Part model, mm, in its own coordinate system. Round coordinates to 2 decimals unless told otherwise and drop trailing zeros. Order: outer loops, then holes, each group sorted by start corner. A loop starts at its lowest first (then second) coordinate and runs counter-clockwise, first axis right, second up. Notation, with made-up numbers: (10.5, 7) -> (43.5, 7) arc R16 ccw to (43.5, 29) -> close; hole circle Ø9 at (15, 2). An arc over 180 degrees is marked (long way). Answer as a JSON object with one key per item and string values. Group by question number.
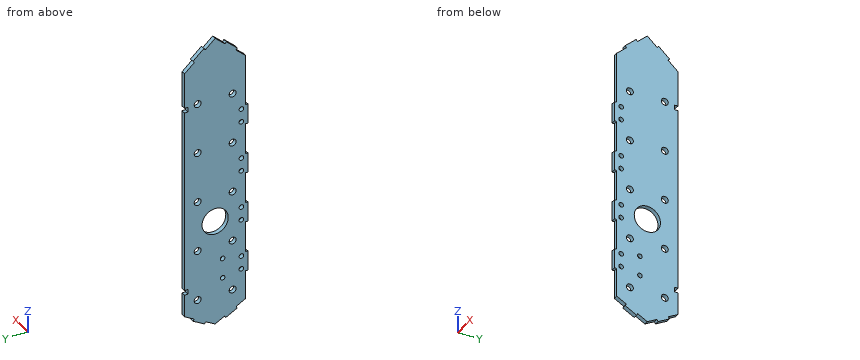
```python
from build123d import *

# Parameters (mm, degrees)
SKETCH1_W                   = 558.8
SKETCH1_H                   = 88.9
BOSS_EXTRUDE1_DEPTH         = 6.35
BOSS_EXTRUDE2_DEPTH         = 6.35
F_3_8_CLEARANCE_HOLE2_D     = 10.0838
F_3_8_CLEARANCE_HOLE3_D     = 10.0838
F_3_8_CLEARANCE_HOLE3_DEPTH = 12.7
F_3_8_CLEARANCE_HOLE3_TIP   = 3.029479155
SKETCH9_W                   = 239.47208483
SKETCH9_H                   = 88.9
CUT_EXTRUDE1_DEPTH          = 322.947408556
BOSS_EXTRUDE3_DEPTH         = 6.35
BOSS_EXTRUDE4_DEPTH         = 6.35
SKETCH12_R                  = 19.05
CUT_EXTRUDE2_DEPTH          = 322.947408556
SKETCH13_W                  = 6.858
SKETCH13_H                  = 5.2705
SKETCH13_W_2                = 6.35
SKETCH13_H_2                = 4.7625
CUT_EXTRUDE3_DEPTH          = 322.947408556
F_1_4_CLEARANCE_HOLE1_D     = 6.7564
F_1_4_CLEARANCE_HOLE2_D     = 6.7564
SKETCH18_W                  = 28.575
SKETCH18_H                  = 3.175
BOSS_EXTRUDE5_DEPTH         = 6.35


with BuildPart() as part:
    # Sketch1 → Boss-Extrude1 (new body)
    with BuildSketch(Plane(origin=(0, 0, 0), x_dir=(0, 0, -1), z_dir=(1, 0, 0))):
        Rectangle(SKETCH1_W, SKETCH1_H)
    extrude(amount=BOSS_EXTRUDE1_DEPTH)

    # Sketch2 → Boss-Extrude2 (add)
    with BuildSketch(Plane(origin=(6.35, 0, 0), x_dir=(0, 0, -1), z_dir=(1, 0, 0))):
        Polygon((-279.4, 44.45), (-318.800892213, 0), (-279.4, -44.45), align=None)
        Polygon((279.4, 44.45), (318.800892213, 0), (279.4, -44.45), align=None)
    extrude(amount=-BOSS_EXTRUDE2_DEPTH)

    # 3/8 Clearance Hole2 (through all)
    with Locations(Plane(origin=(6.35, 0, 0), x_dir=(0, 0, -1), z_dir=(1, 0, 0))):
        with Locations((-155.575, -25.4), (-155.575, 25.4), (-228.6, 25.4), (-228.6, -25.4)):
            Hole(F_3_8_CLEARANCE_HOLE2_D / 2)

    # 3/8 Clearance Hole3
    with Locations(Plane.ZY):
        with Locations((-63.5, 25.4), (-63.5, -25.4), (9.525, -25.4), (9.525, 25.4), (82.55, 25.4), (82.55, -25.4)):
            Hole(F_3_8_CLEARANCE_HOLE3_D / 2, depth=F_3_8_CLEARANCE_HOLE3_DEPTH)
            with Locations((0, 0, -(F_3_8_CLEARANCE_HOLE3_DEPTH + F_3_8_CLEARANCE_HOLE3_TIP / 2))):  # 118° drill point
                Cone(0, F_3_8_CLEARANCE_HOLE3_D / 2, F_3_8_CLEARANCE_HOLE3_TIP, mode=Mode.SUBTRACT)

    # Sketch9 → Cut-Extrude1 (cut, through all)
    with BuildSketch(Plane(origin=(6.35, 0, 0), x_dir=(0, 0, -1), z_dir=(1, 0, 0))):
        with Locations((202.286042415, 0)):
            Rectangle(SKETCH9_W, SKETCH9_H)
    extrude(amount=-CUT_EXTRUDE1_DEPTH, mode=Mode.SUBTRACT)

    # Sketch10 → Boss-Extrude3 (add)
    with BuildSketch(Plane(origin=(6.35, 0, 0), x_dir=(0, 0, -1), z_dir=(1, 0, 0))):
        Polygon((82.55, -44.45), (106.963898899, 0), (82.55, 44.45), align=None)
    extrude(amount=-BOSS_EXTRUDE3_DEPTH)

    # Sketch11 → Boss-Extrude4 (add)
    with BuildSketch(Plane.ZY):
        Polygon((-90.1923834, 30.535633289), (-92.975256742, 32.064109969), (-102.104388841, 15.442843391), (-99.321515499, 13.914366711), align=None)
        Polygon((-99.321515499, -13.914366711), (-102.104388841, -15.442843391), (-92.975256742, -32.064109969), (-90.1923834, -30.535633289), align=None)
        Polygon((292.036372489, 30.194313755), (294.412320197, 32.300375837), (308.540467431, 16.361748326), (306.164519724, 14.255686245), align=None)
        Polygon((306.164519724, -14.255686245), (308.540467431, -16.361748326), (294.412320197, -32.300375837), (292.036372489, -30.194313755), align=None)
    extrude(amount=-BOSS_EXTRUDE4_DEPTH)

    # Sketch12 → Cut-Extrude2 (cut, through all)
    with BuildSketch(Plane.ZY):
        with Locations((46.0375, 0)):
            Circle(SKETCH12_R)
    extrude(amount=-CUT_EXTRUDE2_DEPTH, mode=Mode.SUBTRACT)

    # Sketch13 → Cut-Extrude3 (cut, through all)
    with BuildSketch(Plane.ZY):
        with Locations((224.63125, 42.06875)):
            Rectangle(SKETCH13_W, SKETCH13_H)
        with Locations((224.63125, 42.06875)):
            Rectangle(SKETCH13_W_2, SKETCH13_H_2, mode=Mode.SUBTRACT)
        with Locations((-46.83125, 42.06875)):
            Rectangle(SKETCH13_W, SKETCH13_H)
        with Locations((-46.83125, 42.06875)):
            Rectangle(SKETCH13_W_2, SKETCH13_H_2, mode=Mode.SUBTRACT)
    extrude(amount=-CUT_EXTRUDE3_DEPTH, mode=Mode.SUBTRACT)


with BuildPart() as body_2:
    # of the pieces the cut leaves, the one that is kept (cut_extrude3_keep)
    add(part.part.solids().sort_by_distance((6.35, 44.45, 228.06025))[0])

    # 1/4 Clearance Hole1 (through all)
    with Locations(Plane.ZY):
        with Locations((-41.3385, -10.795), (-12.6365, -10.795)):
            Hole(F_1_4_CLEARANCE_HOLE1_D / 2)

    # 1/4 Clearance Hole2 (through all)
    with Locations(Plane.ZY):
        with Locations((-36.5125, -38.1), (-17.4625, -38.1), (36.5125, -38.1), (55.5625, -38.1), (109.5375, -38.1), (128.5875, -38.1), (182.5625, -38.1), (201.6125, -38.1)):
            Hole(F_1_4_CLEARANCE_HOLE2_D / 2)

    # Sketch18 → Boss-Extrude5 (add)
    with BuildSketch(Plane.ZY):
        with Locations((-26.9875, -46.0375)):
            Rectangle(SKETCH18_W, SKETCH18_H)
        with Locations((46.0375, -46.0375)):
            Rectangle(SKETCH18_W, SKETCH18_H)
        with Locations((119.0625, -46.0375)):
            Rectangle(SKETCH18_W, SKETCH18_H)
        with Locations((192.0875, -46.0375)):
            Rectangle(SKETCH18_W, SKETCH18_H)
    extrude(amount=-BOSS_EXTRUDE5_DEPTH)


solid = body_2.part
```
Q1. Drop flat-ended pins along their axis: pin 1 Ø3.5 at (x, y) = (4, -46.5) entering from +Z (3 decimals); pin 2 Ø1 at (x, y) = (4, -22.5) entering from +Z; pin 3 Ø2.5 at (x, y) = (2.5, -45.5) entering from +Z. Give the stop position or say it passes through.
Q2. Band-saw the part on D-D (z = -63). List the corners of the cut face in (x, y), plus the area to 3 significant figures.
Q3. Band-saw the part on C-C (y = -25.4). List the corners of the cut face in (x, z), plus the area to 3 significant figures.
Q4. Band-saw the part on A-A (z = 82.55). List the corners of the cut face in (x, y), plus the area to 3 significant figures.
Q5. Band-saw the part on B-B (y = 7.5). List the corners of the cut face in (x, z), plus the area to 3 significant figures.
Q6. Wall check: line 1 (Y direction, x = 1.5, z = -63.5); line 2 (Z direction, x = 4.25, y = -28.5); line 3 (Y direction, x = 1.5, z = 235). Give the ranges that are in metal, low to high. Write a range as [from, to].
Completed:
{
 "1": {"pin 1": "z = 206.375", "pin 2": "z = 303.54", "pin 3": "z = 279.58"},
 "2": {"outline": "(0, -44.45) -> (6.35, -44.45) -> (6.35, -30.42) -> (0, -30.42) -> close; (0, -20.38) -> (6.35, -20.38) -> (6.35, 20.38) -> (0, 20.38) -> close; (0, 30.42) -> (6.35, 30.42) -> (6.35, 44.45) -> (0, 44.45) -> close", "area": "437 mm2"},
 "3": {"outline": "(0, -96.64) -> (6.35, -96.64) -> (6.35, -68.54) -> (0, -68.54) -> close; (0, -58.46) -> (6.35, -58.46) -> (6.35, 4.48) -> (0, 4.48) -> close; (0, 14.57) -> (6.35, 14.57) -> (6.35, 77.51) -> (0, 77.51) -> close; (0, 87.59) -> (6.35, 87.59) -> (6.35, 150.53) -> (0, 150.53) -> close; (0, 160.62) -> (6.35, 160.62) -> (6.35, 223.56) -> (0, 223.56) -> close; (0, 233.64) -> (6.35, 233.64) -> (6.35, 300.53) -> (0, 300.53) -> close", "area": "2,200 mm2"},
 "4": {"outline": "(0, -44.45) -> (6.35, -44.45) -> (6.35, -30.44) -> (0, -30.44) -> close; (0, -20.36) -> (6.35, -20.36) -> (6.35, 20.36) -> (0, 20.36) -> close; (0, 30.44) -> (6.35, 30.44) -> (6.35, 44.45) -> (0, 44.45) -> close", "area": "436 mm2"},
 "5": {"outline": "(0, -102.84) -> (6.35, -102.84) -> (6.35, 28.53) -> (0, 28.53) -> close; (0, 63.55) -> (6.35, 63.55) -> (6.35, 312.15) -> (0, 312.15) -> close", "area": "2,410 mm2"},
 "6": {"line 1": "[-44.45, -30.44], [-20.36, 20.36], [30.44, 44.45]", "line 2": "[-94.93, -67.48], [-59.52, 5.55], [13.5, 78.57], [86.53, 151.6], [159.55, 224.62], [232.58, 297.78]", "line 3": "[-44.45, 44.45]"}
}
